Geometry: final body of the model. Coordinates: model frame, mm. A direction names the side the tool comes from. Give positions to 0.01 mm unless a question says otherwise; leave off trailing zeros. Write each loop counter-clockwise with the first axis right and the second up, starting at its lowest first coordinate (ties: lowest second). Pieces come first, ordered by that corner, then holes. Notation, with made-up numbers: (80, 3) -> (127, 3) arc R9 cw to (127, 10) -> close; hole circle Ø2 at (-25, 61.5). An arc over 180 degrees is marked (long way). Answer as a JSON object with one key per item and string values.
from build123d import *

# Parameters (mm, degrees)
PAD004_DEPTH      = 90
POCKET_DEPTH      = 4.551
POCKET_DEPTH_BACK = 4.451
SKETCH028_R       = 2.6
PAD011_DEPTH      = 6
POCKET014_DEPTH   = 3
FILLET011_R       = 3


with BuildPart() as part:
    # Sketch008 (on Face1 of CopyFusion010) → Pad004 (new body)
    with BuildSketch(Plane(origin=(-0.05, -99.1, -81.8), x_dir=(0, 0, -1), z_dir=(0, 1, 0))):
        with BuildLine():
            Line((0, -4.5), (-7.555119, -3.18194))
            ThreePointArc((-7.555119, 3.18194), (-10.23, 0), (-7.555119, -3.18194))
            Line((-7.555119, 3.18194), (0, 4.5))
            Line((37.178474, 1.715195), (0, 4.5))
            ThreePointArc((37.178474, -1.715195), (38.77, 0), (37.178474, 1.715195))
            Line((0, -4.5), (37.178474, -1.715195))
        make_face()
    extrude(amount=PAD004_DEPTH)

    # Sketch027 → Pocket (cut, two sides)
    with BuildSketch(Plane.YZ) as pocket_sk:
        Polygon((-9.1, -139.355119), (-41.57038, -139.355119), (-9.1, -89.355119), align=None)
        Polygon((-9.1, -27.8), (-70.1, -27.8), (-19.1, -78.8), (-14.1, -78.8), (-13.1, -77.8), (-9.1, -77.8), align=None)
    extrude(amount=-POCKET_DEPTH, mode=Mode.SUBTRACT)
    extrude(pocket_sk.sketch, amount=POCKET_DEPTH_BACK, mode=Mode.SUBTRACT)

    # Sketch028 (on Face8 of Pocket) → Pad011 (join)
    with BuildSketch(Plane(origin=(-0.05, -9.1, -81.8), x_dir=(0, 0, -1), z_dir=(0, 1, 0))):
        Circle(SKETCH028_R)
    extrude(amount=PAD011_DEPTH)

    # Sketch038 (on Face2 of Pad011) → Pocket014 (cut)
    with BuildSketch(Plane(origin=(-0.05, -99.1, -81.8), x_dir=(0, 0, -1), z_dir=(0, -1, 0))):
        with BuildLine():
            ThreePointArc((1.966812, 3.192828), (-3.75, 0), (1.966812, -3.192828))
            Line((14.142845, -2.495916), (1.966812, -3.192828))
            ThreePointArc((14.142845, -2.495916), (16.5, 0), (14.142845, 2.495916))
            Line((1.966812, 3.192828), (14.142845, 2.495916))
        make_face()
    extrude(amount=-POCKET014_DEPTH, mode=Mode.SUBTRACT)

    # Fillet011
    fillet011_edges = [part.edges().sort_by_distance(p)[0] for p in [
        (3.926622, -16.6, -78.8),
        (-4.026622, -16.6, -78.8),
    ]]
    fillet(fillet011_edges, radius=FILLET011_R)


solid = part.part
Q1. Material intervals for L1, parallel to X at y = -97.3, z = -81.8; L2, parallel to X at y = -83, z = -99; L3, parallel to Y at x = 1.75, z = -89, sorted ascending. Write a range as from..to.
Values:
{"L1": "-4.55..-3.8, 3.7..4.45", "L2": "-3.26..3.16", "L3": "-96.1..-9.1"}
Q2. Set-up query: faces 4 (the flat face through (0, -17, -78.8)), 5 (the cylindrical face through (2.982, -16.635, -79.248)), 6 (the flat face through (2.8, -97.62, -89.77)). Return all of +Z, -Z, +X, -X, +Y, -Y with unobstructed straight access to the full face (end or side cutting, diameter ignored); none if empty.
Values:
{"face 4": "+Z, +X, -X", "face 5": "+Z, +X", "face 6": "-Y"}
Q3. Cut plane A-A (y = -45). Return the cut outline in (x, z), and give its area (3 significant figures).
Values:
{"outline": "(-4.55, -81.8) -> (-1.77, -118.98) arc R1.72 ccw to (1.67, -118.98) -> (4.45, -81.8) -> (3.13, -74.24) arc R3.23 ccw to (-3.23, -74.24) -> close", "area": "306 mm²"}
Q4. First-contact query: P1, Ø3, axis at x = 0.5, y = -42.5, coming from the +Z side; P2, Ø1, axis at y = -32.5, z = -114, coming from the +X side; P3, Ø1.5, axis at y = -70, z = -115, coming from the -X side; P4, Ø2, axis at x = -0.5, y = -10.5, coming from the +Z side. Flat tips, straight axial feed; report the tip coordinate or a pass-through.
Values:
{"P1": "z = -71.57", "P2": "x = 2.08", "P3": "x = -2.12", "P4": "z = -77.8"}
Q5. Mould query, pull axis Z, two halves, no side actions, for faces 1 (the flat face through (-0.1, -13.7, -78.4)), 2 (the cylindrical face through (-0.1, -97.6, -98.3)), 3 (the flat face through (-3.14, -54.73, -100.65)). Classes: pulls with the +Z half, pulls with the -Z half, needs draft (parallel to the pull), parting line crosses it, or undercut.
Values:
{"face 1": "pulls with the +Z half", "face 2": "undercut", "face 3": "pulls with the -Z half"}
Q6. Cut plane B-B (y = -22). Return the cut outline in (x, z).
Values:
{"outline": "(-4.55, -81.8) -> (-2.5, -109.22) -> (2.4, -109.22) -> (4.45, -81.8) -> (3.42, -75.9) -> (-3.52, -75.9) -> close"}
